Input: dimensioned drawing with shaded views. Units: mm. Origin: part minimum x, y, z. A direction names the side the tool comes from. Coordinates: 2 decimals unless noted, no trailing zeros. Loops run counter-clockwise (first coordinate to the right, second up) from the corner with the lowest first, then second, coordinate; pieces in that order, holes last. Notation, with made-up numbers: (65, 79) - (116, 79) arc R34 cw to (116, 109) - close; hole circle Ø7 at (78.5, 60). An arc over 180 degrees is marked (long way). Put each result on its own line as item: value. Start each with the question number.
1) Section B-B on z = 7.75. Output: boundary loops of the cut face in (x, y), and give its area (3 significant figures).
2) Section A-A on x = 9.5. Output: boundary loops of the cut face in (y, z), and give its area (4 significant figures).
3) Section C-C on y = 23. Output: boundary loops of the cut face in (x, z).
4) Material intervals for line 1 along X through (y, z) = (7.25, 18); line 2 along Y through (x, z) = (20.75, 13); line 3 along X through (y, z) = (1.75, 7), sorted ascending. Write a range as from..to.
5) Reachability of the marked faces 1, 2, 3, 4 and 5 from +Z, -Z, +X, -X, +Y, -Y: full face, straight path, thin tool, end or side. Return the list, or none.
6) Draft query along Z for the marked faces 6, 7, 8 and 9. Return one class per face: +Z half, -Z half, draft (parallel to the pull), parting line (faces both ways), or undercut.
7) Section D-D on x = 19. Output: boundary loops of the cut face in (y, z).
8) Contact query for flat-ended pins moving along their axis: pin 1 Ø1.8 at (x, y) = (12, 23.5) entering from -Z; pin 2 Ø1 at (x, y) = (16.5, 17.5) entering from +Z; pin 3 Ø2 at (x, z) = (13, 13) entering from -Y; pin 4 Ø4.5 at (y, z) = (15.5, 16) entering from +X. Output: stop coordinate, or through.
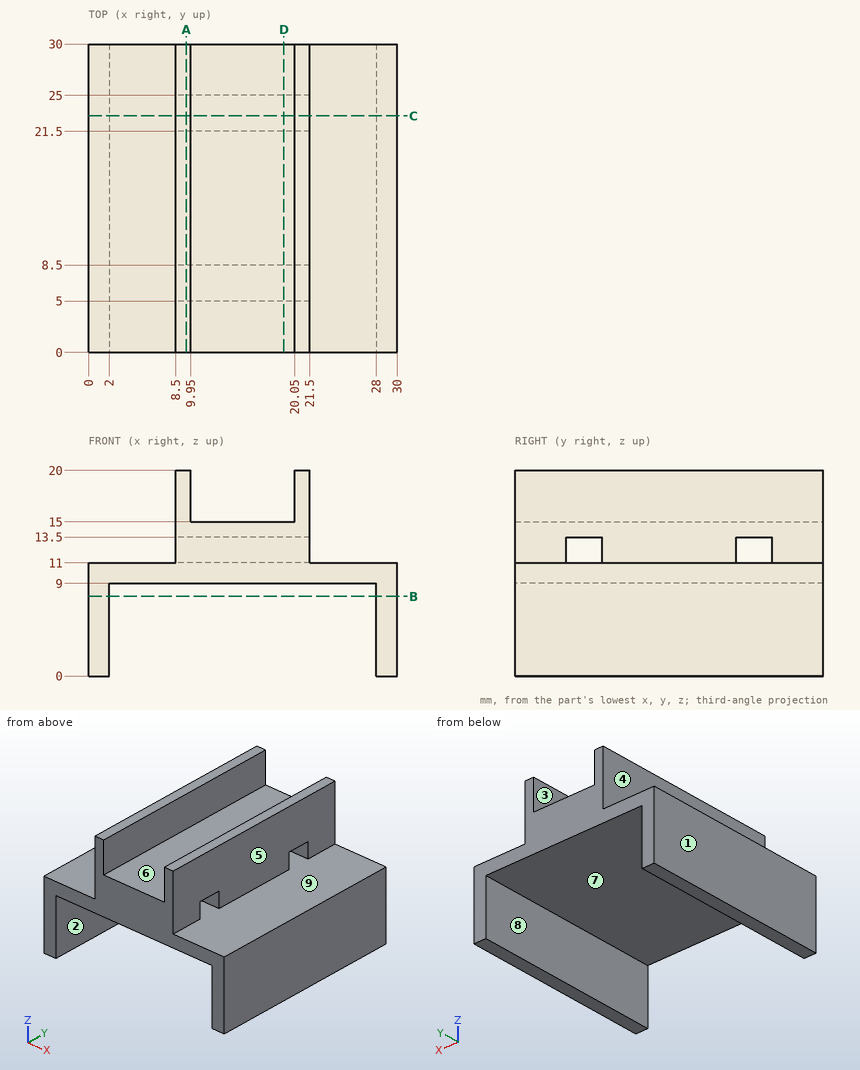
Answer block:
1. outline: (0, 0) - (2, 0) - (2, 30) - (0, 30) - close; (28, 0) - (30, 0) - (30, 30) - (28, 30) - close
1. area: 120 mm²
2. outline: (0, 9) - (30, 9) - (30, 20) - (0, 20) - close; hole (5, 11) - (8.5, 11) - (8.5, 13.5) - (5, 13.5) - close; hole (21.5, 11) - (25, 11) - (25, 13.5) - (21.5, 13.5) - close
2. area: 312.5 mm²
3. outline: (0, 0) - (2, 0) - (2, 9) - (28, 9) - (28, 0) - (30, 0) - (30, 11) - (0, 11) - close; (8.5, 13.5) - (21.5, 13.5) - (21.5, 20) - (20.05, 20) - (20.05, 15) - (9.95, 15) - (9.95, 20) - (8.5, 20) - close
4. line 1: x = 8.5..9.95, 20.05..21.5
4. line 2: y = 0..5, 8.5..21.5, 25..30
4. line 3: x = 0..2, 28..30
5. face 1: +Z, -Z, -X, +Y, -Y
5. face 2: -Z, +Y, -Y
5. face 3: +Z, +Y, -Y
5. face 4: +Z, -X, +Y, -Y
5. face 5: +Z, +X, +Y, -Y
6. face 6: +Z half
6. face 7: -Z half
6. face 8: draft
6. face 9: undercut
7. outline: (0, 9) - (30, 9) - (30, 15) - (0, 15) - close; hole (5, 11) - (8.5, 11) - (8.5, 13.5) - (5, 13.5) - close; hole (21.5, 11) - (25, 11) - (25, 13.5) - (21.5, 13.5) - close
8. pin 1: stops at z = 9
8. pin 2: stops at z = 15
8. pin 3: stops at y = 0
8. pin 4: stops at x = 21.5
